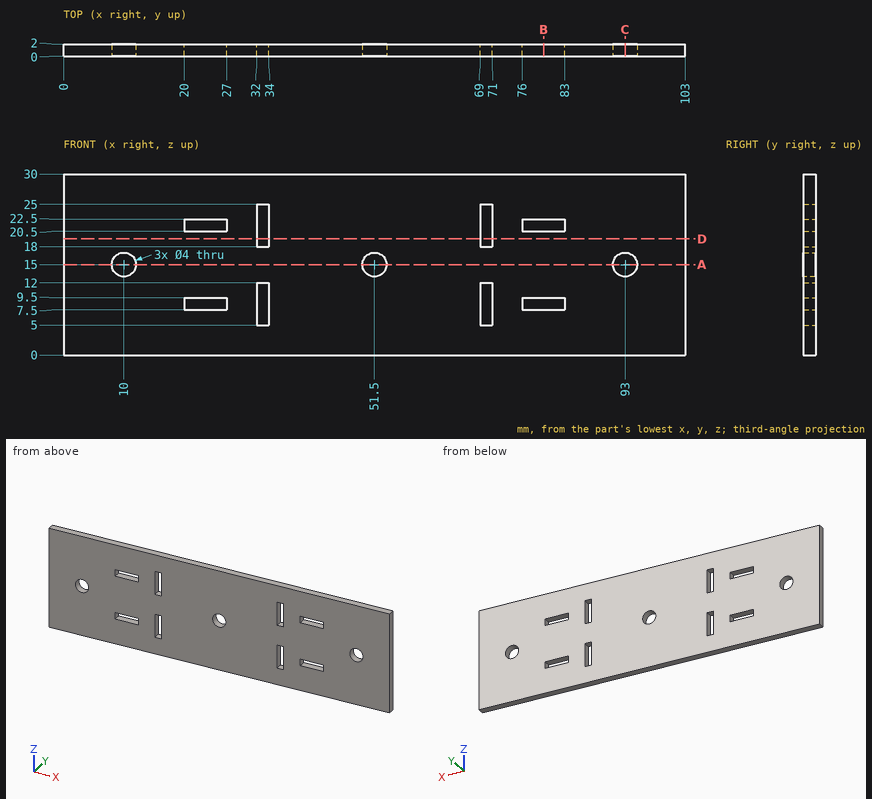
Verification items for this drawing (mm, ordinates from the low corner). Coordinates: 2 decimals unless noted, no trailing zeros. Order: outer loops, then holes, each group sorted by start corner. A loop starts at its lowest first (then second) coordinate and runs counter-clockwise, first axis right, second up. Notation, with made-up numbers: (51, 72.5) -> (78, 72.5) arc R26 ccw to (78, 92.5) -> close; hole circle Ø8 at (8.5, 35.5). An arc over 180 degrees is marked (long way). Put each result on its own line as item: value. Start each with the question number.
1. Cross-section at B-B, the plane x = 79.5. Record the boundary of the cut face in (y, z).
2. Cross-section at D-D, the plane z = 19.25. Record the boundary of the cut face in (x, y), then the cut area to 3 significant figures.
3. Cross-section at C-C, the plane x = 93. Record the boundary of the cut face in (y, z).
4. Material ranges on L1, parallel to Z at x = 23.5, y = 0.2; L2, parallel to X at y = 1.3, z = 15; L3, parallel to X at y = 0.35, z = 6.75, recorded low to high. Write a range as [from, to].
5. Cross-section at A-A, the plane z = 15. Record the boundary of the cut face in (x, y).
Computed:
1. outline: (0, 0) -> (2, 0) -> (2, 7.5) -> (0, 7.5) -> close; (0, 9.5) -> (2, 9.5) -> (2, 20.5) -> (0, 20.5) -> close; (0, 22.5) -> (2, 22.5) -> (2, 30) -> (0, 30) -> close
2. outline: (0, 0) -> (32, 0) -> (32, 2) -> (0, 2) -> close; (34, 0) -> (69, 0) -> (69, 2) -> (34, 2) -> close; (71, 0) -> (103, 0) -> (103, 2) -> (71, 2) -> close
2. area: 198 mm2
3. outline: (0, 0) -> (2, 0) -> (2, 13) -> (0, 13) -> close; (0, 17) -> (2, 17) -> (2, 30) -> (0, 30) -> close
4. L1: [0, 7.5], [9.5, 20.5], [22.5, 30]
4. L2: [0, 8], [12, 49.5], [53.5, 91], [95, 103]
4. L3: [0, 32], [34, 69], [71, 103]
5. outline: (0, 0) -> (8, 0) -> (8, 2) -> (0, 2) -> close; (12, 0) -> (49.5, 0) -> (49.5, 2) -> (12, 2) -> close; (53.5, 0) -> (91, 0) -> (91, 2) -> (53.5, 2) -> close; (95, 0) -> (103, 0) -> (103, 2) -> (95, 2) -> close
